Model file for the job. Use its own axes, mm. Give positions to 0.01 mm unless a question says otherwise; leave off trailing zeros. Order: outer loops, then holes, each group sorted by start corner. A loop starts at its lowest first (then second) coordinate and runs counter-clockwise, first axis right, second up. Notation, with made-up numbers: (88, -4.5) - (115, -4.5) arc R20 ccw to (115, 1.5) - close; hole circle Ø10 at (61.25, -13). An arc over 180 degrees is marked (long way). Return JSON: item names as keys, results as strings. Group by question number.
from build123d import *

# Parameters (mm, degrees)
PAD_DEPTH    = 1.5
CHAMFER_SIZE = 0.749


with BuildPart() as part:
    # Sketch → Pad (new body)
    with BuildSketch(Plane.XZ):
        Polygon((-8, 4), (-8, -2.5), (-4, -4), (4, -4), (8, -2.5), (8, 4), align=None)
    extrude(amount=PAD_DEPTH)

    # Chamfer
    chamfer_edges = [part.edges().sort_by_distance(p)[0] for p in [
        (0, -1.5, -4),
        (0, 0, -4),
    ]]
    chamfer(chamfer_edges, length=CHAMFER_SIZE)


solid = part.part
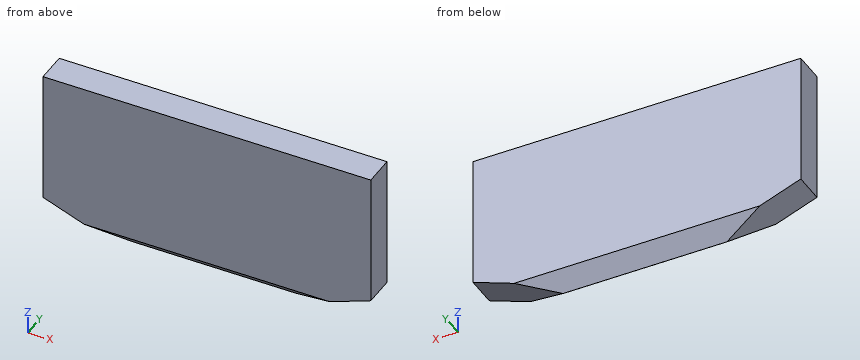
(1) Slice it at C-C (z = -3). Give the cut face in (x, y).
(2) Drill centre lines: L1, parallel to Z at x = -1.5, y = -0.9; L2, parallel to Z at x = -5.5, y = -0.3. Where is each one in solid material? Low to high.
(3) Slice it at B-B (y = -0.5). Give the cut face in (x, z), and give its area (3 significant figures).
Result set:
{
 "1": {"outline": "(-6.67, -1.5) - (6.67, -1.5) - (6.67, 0) - (-6.67, 0) - close"},
 "2": {"L1": "z = -3.85 to 4", "L2": "z = -3.44 to 4"},
 "3": {"outline": "(-8, -2.5) - (-4.66, -3.75) - (4.66, -3.75) - (8, -2.5) - (8, 4) - (-8, 4) - close", "area": "120 mm²"}
}
